Work out the finished part from the listing and answer in its coordinate system (mm). A direction names the side the tool comes from. Coordinates: 2 decimals unless noted, no trailing zeros. Order: outer loops, then holes, each group sorted by start corner. A loop starts at its lowest first (then second) coordinate and runs counter-clockwise, first axis right, second up. Notation, with made-up numbers: M 70.25,-30 L 112.25,-30 A18 cw 112.25,-25 Z; hole C -33.75,-26 d9. An arc over 180 degrees is marked long. Answer in a Markdown table with one row per item. Add a question column.
Item 1: The part is cut by section B-B (y = 0.4). Write down the section's boundary in (x, z), then the cut area to 3 significant figures.
Item 2: A flat-ended cylindrical pin translates along its axis: pin 1 Ø0.8 at (x, y) = (-2.5, 0.5) entering from -Z. Find the tip coordinate at first contact, or state that the pin passes through.
Item 3: The part is cut by section A-A (z = 0). Write down the section's boundary in (x, y).
Item 4: The part is cut by section C-C (x = 8.5). Write down the section's boundary in (y, z), then the cut area to 4 significant figures.
Item 5: Which of the six approach directions +Z, -Z, +X, -X, +Y, -Y give full straight-line access (tool end or side, diameter ignored) to faces 1 (the face through (14.05, 0.49, 0.05)), 2 (the face through (0.2, 0.5, -2.45)), 3 (the face through (-14.05, 0.49, -0.05)), 4 (the face through (-0.2, 0.5, 2.45))?
Item 6: The mould has two halves that part along Z. Classify faces 5 (the face through (15.25, -0.25, 0.08)), 6 (the face through (-10.46, 0.01, -0.15)), 7 (the face through (12.74, 0.01, -0.15)), 8 (the face through (0, 0, -3)): released by +Z, released by -Z, zero draft, split by the parting line, or undercut.
Item 7: Consider line 1 (X direction, y = 0.1, z = 0); line 2 (X direction, y = -0.45, z = 0); line 3 (Y direction, x = 4, z = 2.75). Determine where each line is inside the solid, lowest interval first. Write a range as from..to.
from build123d import *

# Parameters (mm, degrees)
BOSS_EXTRUDE1_DEPTH = 1
BOSS_EXTRUDE2_DEPTH = 1
SKETCH4_R           = 1.15
CUT_EXTRUDE1_DEPTH  = 16.807751263
CHAMFER1_SIZE       = 0.5


with BuildPart() as part:
    # Sketch2 → Boss-Extrude1 (new body)
    with BuildSketch(Plane(origin=(0, 0, 0), x_dir=(1, 0, 0), z_dir=(0, 1, 0))):
        with BuildLine():
            Line((11.6, 3.65), (-11.6, 3.65))
            ThreePointArc((-11.6, 3.65), (-15.25, 0), (-11.6, -3.65))
            Line((-11.6, -3.65), (11.6, -3.65))
            ThreePointArc((11.6, -3.65), (15.25, 0), (11.6, 3.65))
        make_face()
    extrude(amount=-BOSS_EXTRUDE1_DEPTH)

    # Sketch3 → Boss-Extrude2 (add)
    with BuildSketch(Plane(origin=(0, 0, 0), x_dir=(1, 0, 0), z_dir=(0, 1, 0))):
        with BuildLine():
            Line((-11.6, -2.45), (11.6, -2.45))
            ThreePointArc((11.6, -2.45), (14.05, 0), (11.6, 2.45))
            Line((11.6, 2.45), (-11.6, 2.45))
            ThreePointArc((-11.6, 2.45), (-14.05, 0), (-11.6, -2.45))
        make_face()
    extrude(amount=BOSS_EXTRUDE2_DEPTH)

    # Sketch4 → Cut-Extrude1 (cut, through all)
    with BuildSketch(Plane(origin=(0, 1, 0), x_dir=(1, 0, 0), z_dir=(0, 1, 0))):
        with Locations(Location((-11.6, 0, 0), (0, 0, 270))):
            Circle(SKETCH4_R)
        with Locations(Location((11.6, 0, 0), (0, 0, 270))):
            Circle(SKETCH4_R)
    extrude(amount=-CUT_EXTRUDE1_DEPTH, mode=Mode.SUBTRACT)

    # Chamfer1
    chamfer1_edges = [part.edges().sort_by_distance(p)[0] for p in [
        (15.25, -1, 0),
        (0, -1, -3.65),
        (-15.25, -1, 0),
        (0, -1, 3.65),
    ]]
    chamfer(chamfer1_edges, length=CHAMFER1_SIZE)


solid = part.part
Reply:
| question | item | result |
|---|---|---|
| 1 | outline | M -11.6,-2.45 L 11.6,-2.45 A2.45 ccw 11.6,2.45 L -11.6,2.45 A2.45 ccw Z; hole C -11.6,0 d2.3; hole C 11.6,0 d2.3 |
| 1 | area | 124 mm2 |
| 2 | pin 1 | stops at z = -2.45 |
| 3 | outline | M -15.25,-0.5 L -14.75,-1 L -12.75,-1 L -12.75,1 L -14.05,1 L -14.05,0 L -15.25,0 Z; M -10.45,-1 L 10.45,-1 L 10.45,1 L -10.45,1 Z; M 12.75,-1 L 14.75,-1 L 15.25,-0.5 L 15.25,0 L 14.05,0 L 14.05,1 L 12.75,1 Z |
| 4 | outline | M -1,-3.15 L -0.5,-3.65 L 0,-3.65 L 0,-2.45 L 1,-2.45 L 1,2.45 L 0,2.45 L 0,3.65 L -0.5,3.65 L -1,3.15 Z |
| 4 | area | 11.95 mm2 |
| 5 | face 1 | +X, +Y |
| 5 | face 2 | -Z, +X, -X, +Y |
| 5 | face 3 | -X, +Y |
| 5 | face 4 | +Z, +X, -X, +Y |
| 6 | face 5 | split by the parting line |
| 6 | face 6 | undercut |
| 6 | face 7 | undercut |
| 6 | face 8 | zero draft |
| 7 | line 1 | x = -14.05..-12.75, -10.45..10.45, 12.75..14.05 |
| 7 | line 2 | x = -15.25..-12.75, -10.45..10.45, 12.75..15.25 |
| 7 | line 3 | y = -1..0 |
